Design review of the part built by this model. Coordinates are the model's own, in mm. Face numbers are marked on the shaded views. A direction names the side the tool comes from. Round coordinates to 2 decimals unless told otherwise and drop trailing zeros. Write each loop counter-clockwise with the first axis right and the second up, starting at its lowest first coordinate (ties: lowest second). Pieces come first, ordered by that corner, then holes. Notation, with made-up numbers: M 86,3.25 L 95,3.25 A24 cw 95,34.25 Z; hole C 52.25,1 d11. An arc over 180 degrees is marked long. Use CSV: the item, a comma, the result in double quotes.
from build123d import *

# Parameters (mm, degrees)
F0_W      = 36
F0_H      = 24
F1_DEPTH  = 18
F5_W      = 36
F5_H      = 36
F5_R      = 16
F6_DEPTH  = 2
F8_R      = 16.5
F8_R_2    = 16
F9_DEPTH  = 2
F10_R     = 2
F2_R      = 1.25
F13_DEPTH = 36.001
F3_R      = 1.25
F14_DEPTH = 36.001
F4_R      = 1.25
F15_DEPTH = 3
F7_R      = 1.25
F16_DEPTH = 3


# Not quite as in the source:
# - a feature of the source that left no trace in its solid (it failed there, or was rolled back) is left out


with BuildPart() as f1:
    # F0 (on Right) → F1 (new body, symmetric)
    with BuildSketch(Plane.YZ):
        Rectangle(F0_W, F0_H)
    extrude(amount=F1_DEPTH, both=True)

    # F5 (on face) → F6 (cut)
    with BuildSketch(Plane.XY.offset(12)):
        Rectangle(F5_W, F5_H)
        Circle(F5_R, mode=Mode.SUBTRACT)
    extrude(amount=-F6_DEPTH, mode=Mode.SUBTRACT)

    # F8 (on face) → F9 (cut)
    with BuildSketch(Plane.XY.offset(10)):
        Circle(F8_R)
        Circle(F8_R_2, mode=Mode.SUBTRACT)
    extrude(amount=-F9_DEPTH, mode=Mode.SUBTRACT)

    # F10
    f10_edges = [f1.edges().sort_by_distance(p)[0] for p in [
        (-18, -18, -1),
        (-18, 18, -1),
        (18, -18, -1),
        (-18, 0, -12),
        (0, 18, -12),
        (18, 0, -12),
        (0, -18, -12),
        (18, 18, -1),
    ]]
    fillet(f10_edges, radius=F10_R)

    # F2 (on face) → F13 (cut, through all)
    with BuildSketch(Plane.XZ.offset(18)):
        with Locations((-12, 6)):
            Circle(F2_R)
        with Locations((12, 6)):
            Circle(F2_R)
        Circle(F2_R)
        with Locations((-12, -6)):
            Circle(F2_R)
        with Locations((12, -6)):
            Circle(F2_R)
    extrude(amount=-F13_DEPTH, mode=Mode.SUBTRACT)

    # F3 (on face) → F14 (cut, through all)
    with BuildSketch(Plane(origin=(-18, 0, 0), x_dir=(0, -1, 0), z_dir=(-1, 0, 0))):
        with Locations((-12, 6)):
            Circle(F3_R)
        with Locations((-12, -6)):
            Circle(F3_R)
        Circle(F3_R)
        with Locations((12, -6)):
            Circle(F3_R)
        with Locations((12, 6)):
            Circle(F3_R)
    extrude(amount=-F14_DEPTH, mode=Mode.SUBTRACT)

    # F4 (on face) → F15 (cut)
    with BuildSketch(Plane.XY.offset(12)):
        with Locations((12, 0)):
            Circle(F4_R)
        with Locations((8.4852813742, 8.4852813742)):
            Circle(F4_R)
        with Locations((0, 12)):
            Circle(F4_R)
        with Locations((-8.4852813742, 8.4852813742)):
            Circle(F4_R)
        with Locations((-12, 0)):
            Circle(F4_R)
        with Locations((-8.4852813742, -8.4852813742)):
            Circle(F4_R)
        with Locations((0, -12)):
            Circle(F4_R)
        with Locations((8.4852813742, -8.4852813742)):
            Circle(F4_R)
    extrude(amount=-F15_DEPTH, mode=Mode.SUBTRACT)

    # F7 (on face) → F16 (cut)
    with BuildSketch(Plane(origin=(0, 0, -12), x_dir=(1, 0, 0), z_dir=(0, 0, -1))):
        with Locations((-12, -12)):
            Circle(F7_R)
        with Locations((-12, 12)):
            Circle(F7_R)
        Circle(F7_R)
        with Locations((12, -12)):
            Circle(F7_R)
        with Locations((12, 12)):
            Circle(F7_R)
    extrude(amount=-F16_DEPTH, mode=Mode.SUBTRACT)


solid = f1.part
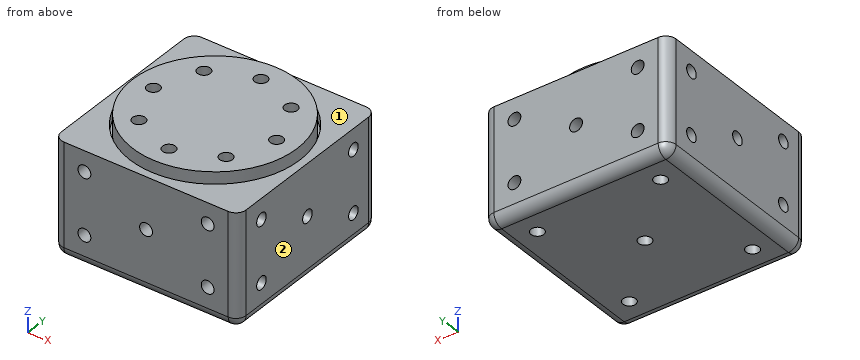
1) Add section D-D on x = 8.5. Write out the cut boundary in (y, z).
Answers:
outline,"M -18,-10 A2 ccw -16,-12 L 16,-12 A2 ccw 18,-10 L 18,10 L 14.14,10 L 14.14,8 L 13.56,8 L 13.56,12 L 9.74,12 L 9.74,9 L 7.24,9 L 7.24,12 L -7.24,12 L -7.24,9 L -9.74,9 L -9.74,12 L -13.56,12 L -13.56,8 L -14.14,8 L -14.14,10 L -18,10 Z; hole C -12,-6 d2.5; hole C -12,6 d2.5; hole C 0,0 d2.5; hole C 12,-6 d2.5; hole C 12,6 d2.5"
2) Add section A-A on z = 0. Write out the cut boundary in (x, y).
Answers:
outline,"M -18,-16 A2 ccw -16,-18 L -1.25,-18 L -1.25,-1.25 L -18,-1.25 Z; M -18,1.25 L -1.25,1.25 L -1.25,18 L -16,18 A2 ccw -18,16 Z; M 1.25,-18 L 16,-18 A2 ccw 18,-16 L 18,-1.25 L 1.25,-1.25 Z; M 1.25,1.25 L 18,1.25 L 18,16 A2 ccw 16,18 L 1.25,18 Z"
3) For pin 1 Ø3 at (x, z) = (-12, 6) entering from -Y; pin 2 Ø1.5 at (x, y) = (-12, 12) entering from -Z, all flat-tipped, find the tip position at first contact; note any pin that passes through.
Answers:
pin 1,"y = -18"
pin 2,"z = -9"
4) Add section B-B on z = 6. Give the number of separate pieces and of enclosed holes in the cut face, then the cut area to 3 significant figures.
Answers:
separate pieces,"9"
enclosed holes,"0"
area,"958 mm²"
5) Machinability: for the marked faces 1 and 2, which of the approach directions +Z, -Z, +X, -X, +Y, -Y give a long, thin tool a straight path to every point of the face, cutting with its end or side? Answer none if there is none.
Answers:
face 1,"+Z"
face 2,"+Z, -Z, +X, +Y, -Y"
6) Wall thickness on line 1 along Y through (x, z) = (-14.55, -6); line 2 along Z through (x, y) = (-12, 14.5): over which ranges is each line inside the solid? List them lowest first. Write a range as [from, to].
Answers:
line 1,"[-18, -13.25], [-10.75, 10.75], [13.25, 18]"
line 2,"[-12, -7.25], [-4.75, 4.75], [7.25, 10]"
